from build123d import *

# Parameters (mm, degrees)
F0_R          = 3
F1_DEPTH      = 35
F2_SIZE       = 0.5
F3_W          = 14.1636701301
F3_H          = 25.4946053028
F4_DEPTH      = 25
F4_DEPTH_BACK = 25
F6_DEPTH      = 25
F6_TAPER      = -8


with BuildPart() as f1:
    # F0 (on Top) → F1 (new body)
    with BuildSketch(Plane.XY):
        Circle(F0_R)
    extrude(amount=F1_DEPTH)

    # F2
    f2_edges = [f1.edges().sort_by_distance(p)[0] for p in [
        (-3, 0, 35),
    ]]
    chamfer(f2_edges, length=F2_SIZE)

    # F3 (on Right) → F4 (cut, two sides)
    with BuildSketch(Plane.YZ) as f4_sk:
        with Locations((-7.081835065, -4.5323744416)):
            Rectangle(F3_W, F3_H)
    extrude(amount=-F4_DEPTH, mode=Mode.SUBTRACT)
    extrude(f4_sk.sketch, amount=F4_DEPTH_BACK, mode=Mode.SUBTRACT)

    # F5 (on Front) → F6 (cut)
    with BuildSketch(Plane.XZ):
        Polygon((30.5935237557, -28.8938842714), (30.5935237557, 13.8803962618), (-26.6276989132, -8.9460639283), (-26.6276989132, -10.4811154306), align=None)
    extrude(amount=-F6_DEPTH, taper=F6_TAPER, mode=Mode.SUBTRACT)


solid = f1.part
Here's how the part is built. I have some questions about the finished solid (model axes, mm). A direction names the side the tool comes from. Round coordinates to 2 decimals unless told otherwise and drop trailing zeros. Loops run counter-clockwise (first coordinate to the right, second up) from the corner with the lowest first, then second, coordinate; pieces in that order, holes last. Notation, with made-up numbers: (3.25, -38.75) - (53.25, -38.75) arc R26 cw to (53.25, -22.75) - close; hole circle Ø11 at (49, 80). An arc over 180 degrees is marked (long way). One line per question, with ' | ' between items. Start each with the question number.
Q1. Will these pins go through, and if not, where does the flat tip stop? pin 1 (1 mm diameter, centred on x = -0.5, y = 0.5, fed in from -Z); pin 2 (1 mm diameter, centred on x = -2, y = 2.5, fed in from -Z); pin 3 (1.5 mm diameter, centred on x = -1, z = 22.5, fed in from -Y).
Q2. For faces 1 (the flat face through (0, -1, 8.215)), 2 (the flat face through (0, 0, 35)), which set-ups out of +Z, -Z, +X, -X, +Y, -Y let a thin tool reach every point of the face, with its end or its side?
Q3. Please list where these lines run through material, in increasing order: line 1 (Z direction, x = 1.5, y = -1.5); line 2 (Z direction, x = -2, y = 1); line 3 (Y direction, x = -2, z = 29.5). Write a range as [from, to].
Q4. I want a section at A-A (z = 8.5). Write out the boundary of the cut face in (x, y).
Response values:
1) pin 1: stops at z = 1.34 | pin 2: stops at z = 1.11 | pin 3: stops at y = -2.99
2) face 1: -Z, +X, -X, -Y | face 2: +Z, +X, -X, +Y, -Y
3) line 1: z = [8.21, 35] | line 2: z = [1.03, 35] | line 3: y = [-2.24, 2.24]
4) outline: circle Ø6 at (0, 0)
